from build123d import *

# Parameters (mm, degrees)
F1_DEPTH = 0.254


with BuildPart() as f1:
    # F0 (on Top) → F1 (new body)
    with BuildSketch(Plane.XY):
        with BuildLine():
            Line((8.255, 12.7), (-8.255, 12.7))
            Line((-8.255, 12.7), (-8.255, 11.43))
            ThreePointArc((-8.255, 11.43), (-4.271494, 11.989244), (-0.254, 12.191285))
            Line((-0.254, 12.191285), (-0.254, 0.254))
            Line((-0.254, 0.254), (-7.746982, 0.254))
            ThreePointArc((-7.746982, 0.254), (-7.554177, 4.06437), (-6.985, 7.83692))
            Line((-6.985, 7.83692), (-8.255, 7.83692))
            Line((-8.255, 7.83692), (-8.255, -7.40308))
            Line((-8.255, -7.40308), (-6.985, -7.40308))
            ThreePointArc((-6.985, -7.40308), (-7.53188, -3.846307), (-7.744118, -0.254))
            Line((-7.744118, -0.254), (-0.254, -0.254))
            Line((-0.254, -0.254), (-0.254, -12.191285))
            ThreePointArc((-0.254, -12.191285), (-4.271494, -11.989244), (-8.255, -11.43))
            Line((-8.255, -11.43), (-8.255, -12.7))
            Line((-8.255, -12.7), (8.255, -12.7))
            Line((8.255, -12.7), (8.255, -11.43))
            ThreePointArc((8.255, -11.43), (4.271494, -11.989244), (0.254, -12.191285))
            Line((0.254, -12.191285), (0.254, -0.254))
            Line((0.254, -0.254), (7.744118, -0.254))
            ThreePointArc((7.744118, -0.254), (7.53188, -3.846307), (6.985, -7.40308))
            Line((6.985, -7.40308), (8.255, -7.40308))
            Line((8.255, -7.40308), (8.255, 7.83692))
            Line((8.255, 7.83692), (6.985, 7.83692))
            ThreePointArc((6.985, 7.83692), (7.554177, 4.06437), (7.746982, 0.254))
            Line((7.746982, 0.254), (0.254, 0.254))
            Line((0.254, 0.254), (0.254, 12.191285))
            ThreePointArc((0.254, 12.191285), (4.271494, 11.989244), (8.255, 11.43))
            Line((8.255, 11.43), (8.255, 12.7))
        make_face()
    extrude(amount=F1_DEPTH)


solid = f1.part
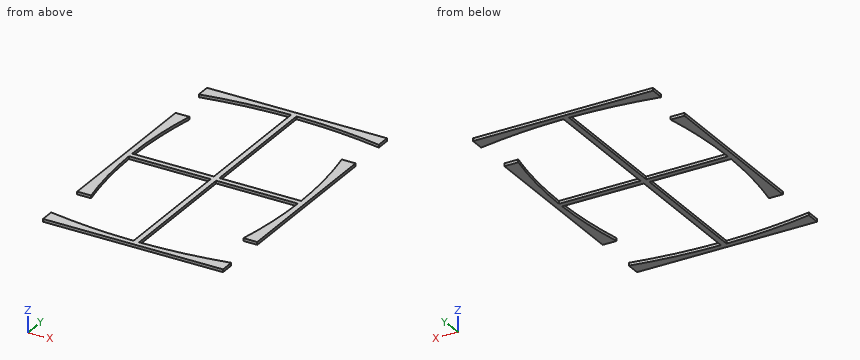
Work out the finished part from the listing and answer in its coordinate system (mm). Coordinates: 2 decimals unless noted, no trailing zeros. Write each loop counter-clockwise with the first axis right and the second up, starting at its lowest first coordinate (ties: lowest second). Pieces come first, ordered by that corner, then holes.
1. The part is cut by section A-A, the plane x = -6.25. Write down the section's boundary in (y, z), and give its area (3 significant figures).
Results list:
outline: (-12.7, 0) - (-11.76, 0) - (-11.76, 0.25) - (-12.7, 0.25) - close; (-0.25, 0) - (0.25, 0) - (0.25, 0.25) - (-0.25, 0.25) - close; (11.76, 0) - (12.7, 0) - (12.7, 0.25) - (11.76, 0.25) - close
area: 0.608 mm2
2. The part is cut by section C-C, the plane z = 0.15. Write down the section's boundary in (x, y) (3 decimals), and give its area (3 significant figures).
Results list:
outline: (-8.255, -12.7) - (8.255, -12.7) - (8.255, -11.43) arc R45.096 cw to (0.254, -12.191) - (0.254, -0.254) - (7.744, -0.254) arc R38.481 cw to (6.985, -7.403) - (8.255, -7.403) - (8.255, 7.837) - (6.985, 7.837) arc R38.481 cw to (7.747, 0.254) - (0.254, 0.254) - (0.254, 12.191) arc R45.096 cw to (8.255, 11.43) - (8.255, 12.7) - (-8.255, 12.7) - (-8.255, 11.43) arc R45.096 cw to (-0.254, 12.191) - (-0.254, 0.254) - (-7.747, 0.254) arc R38.481 cw to (-6.985, 7.837) - (-8.255, 7.837) - (-8.255, -7.403) - (-6.985, -7.403) arc R38.481 cw to (-7.744, -0.254) - (-0.254, -0.254) - (-0.254, -12.191) arc R45.096 cw to (-8.255, -11.43) - close
area: 68.3 mm2
3. Consider line 1 along X through (y, z) = (3.5, 0.2) (3 decimals); line 2 along X through (y, z) = (1.25, 0.15) (3 decimals); line 3 along Y through (x, z) = (5.5, 0.15). Determine where each line is inside the solid, lowest interval first.
Results list:
line 1: x = -8.255 to -7.607, -0.254 to 0.254, 7.607 to 8.255
line 2: x = -8.255 to -7.733, -0.254 to 0.254, 7.733 to 8.255
line 3: y = -12.7 to -11.86, -0.25 to 0.25, 11.86 to 12.7
4. The part is cut by section D-D, the plane y = -7.75. Write down the section's boundary in (x, z).
Results list:
outline: (-0.25, 0) - (0.25, 0) - (0.25, 0.25) - (-0.25, 0.25) - close
5. The part is cut by section B-B, the plane y = -4.25. Write down the section's boundary in (x, z) (3 decimals).
Results list:
outline: (-8.255, 0) - (-7.487, 0) - (-7.487, 0.254) - (-8.255, 0.254) - close; (-0.254, 0) - (0.254, 0) - (0.254, 0.254) - (-0.254, 0.254) - close; (7.487, 0) - (8.255, 0) - (8.255, 0.254) - (7.487, 0.254) - close
